Design review of the part shown in the three views and the two pictorial views. Dimensions are in mm from the part's minimum x, y and z. A direction names the side the tool comes from. Coordinates: 2 decimals unless noted, no trailing zeros. Loops run counter-clockwise (first coordinate to the right, second up) from the corner with the lowest first, then second, coordinate; pieces in that order, holes last.
Q1. Add section C-C on z = 8.25. Give the number of separate pieces and of enclosed holes in the cut face, and give its area (3 significant figures).
Q2. Wall thickness on probe 1 along X at (y, z) = (19.05, 7.75); probe 2 along Y at (x, z) = (9, 11) (1 decimal); probe 3 along X at (y, z) = (17, 7.25) (1 decimal): over which ranges is each line inside the solid? List them lowest first.
Q3. Add section B-B on x = 35. Give the boundary of the cut face in (y, z), and give its area (3 significant figures).
Q4. Add section D-D on y = 127. Give the boundary of the cut face in (x, z).
Q5. Add section A-A on y = 19.05. Give the boundary of the cut face in (x, z).
Q6. For P1, Ø4, axis at x = 28.575, y = 19.05, coming from the -Z side; P2, Ø7.5, axis at x = 9.525, y = 133.604, coming from the -Z side; P3, Ø1, axis at x = 9, y = 97, coming from the -Z side, all flat-tipped, find the tip position at first contact; note any pin that passes through.
Q7. Machinability: for the marked faces 1 and 2, which of the approach directions +Z, -Z, +X, -X, +Y, -Y give a long, thin tool a straight path to every point of the face, cutting with its end or side? Answer none if there is none.
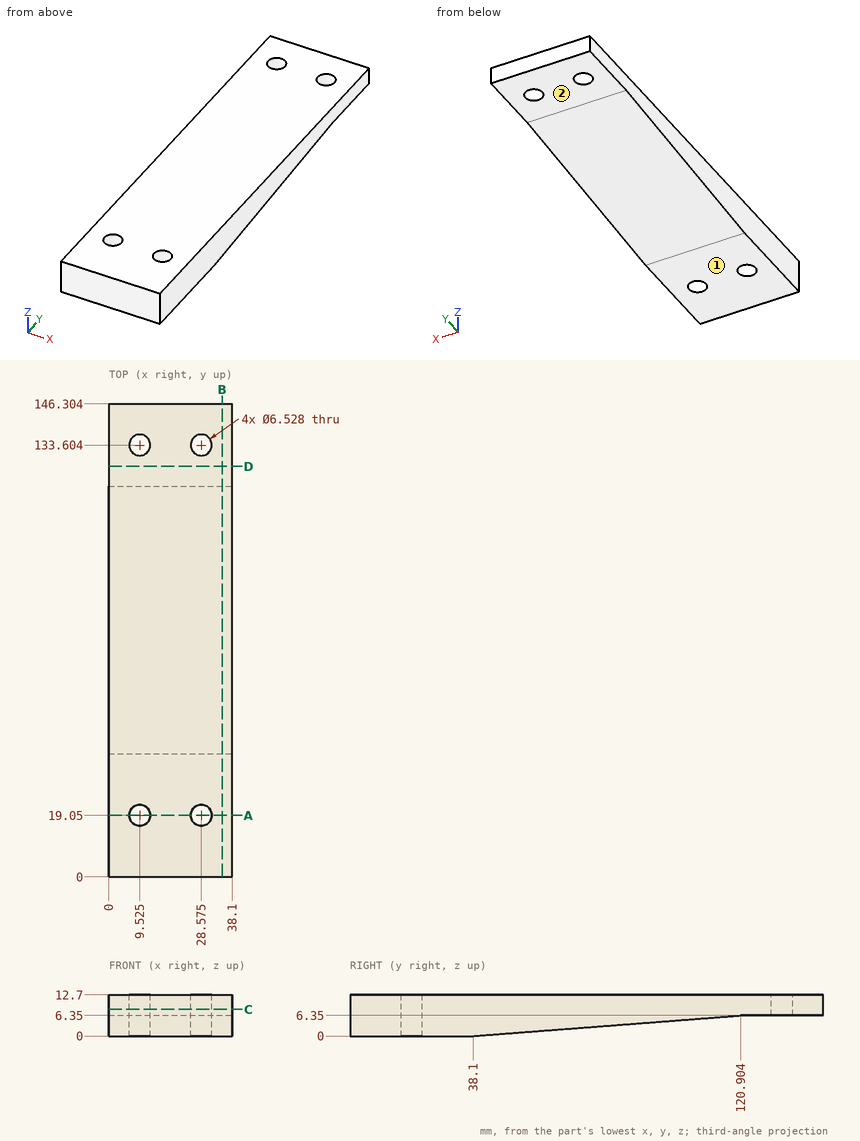
Entries:
1. separate pieces: 1
1. enclosed holes: 4
1. area: 5,440 mm2
2. probe 1: x = 0 to 6.26, 12.79 to 25.31, 31.84 to 38.1
2. probe 2: y = 0 to 15.8, 22.3 to 130.4, 136.8 to 146.3
2. probe 3: x = 0 to 7, 12.1 to 26, 31.1 to 38.1
3. outline: (0, 0) - (38.1, 0) - (120.9, 6.35) - (146.3, 6.35) - (146.3, 12.7) - (0, 12.7) - close
3. area: 1,430 mm2
4. outline: (0, 6.35) - (38.1, 6.35) - (38.1, 12.7) - (0, 12.7) - close
5. outline: (0, 0) - (6.26, 0) - (6.26, 12.7) - (0, 12.7) - close; (12.79, 0) - (25.31, 0) - (25.31, 12.7) - (12.79, 12.7) - close; (31.84, 0) - (38.1, 0) - (38.1, 12.7) - (31.84, 12.7) - close
6. P1: passes through
6. P2: stops at z = 6.35
6. P3: stops at z = 4.48
7. face 1: -Z, +X, -X, +Y, -Y
7. face 2: -Z, +X, -X, +Y
